from build123d import *

# Parameters (mm, degrees)
F0_W     = 60.3283978999
F0_H     = 56.9055080414
F1_DEPTH = 25.4
F3_DEPTH = 5.08
F5_DEPTH = 25.401


with BuildPart() as f1:
    # F0 (on Top) → F1 (new body)
    with BuildSketch(Plane.XY):
        with Locations((30.1641989499, 28.4527540207)):
            Rectangle(F0_W, F0_H)
    extrude(amount=F1_DEPTH)

    # F2 (on face) → F3 (cut)
    with BuildSketch(Plane.XY.offset(25.4)):
        with BuildLine():
            ThreePointArc((55.1804514534, 39.8446242733), (55.3108318877, 40.8708207203), (55.3543950429, 41.9043488801))
            ThreePointArc((55.3543950429, 41.9043488801), (36.2534657798, 52.11936711), (38.3624892299, 30.5614424362))
            ThreePointArc((38.3624892299, 30.5614424362), (42.0828202021, 43.6972697394), (55.1804514534, 39.8446242733))
        make_face()
        with BuildLine():
            ThreePointArc((55.1804514534, 39.8446242733), (42.0828202021, 43.6972697394), (38.3624892299, 30.5614424362))
            ThreePointArc((38.3624892299, 30.5614424362), (49.0077038635, 31.1517402149), (55.1804514534, 39.8446242733))
        make_face()
        with BuildLine():
            ThreePointArc((55.1804514534, 39.8446242733), (49.0077038635, 31.1517402149), (38.3624892299, 30.5614424362))
            ThreePointArc((38.3624892299, 30.5614424362), (49.1682517649, 25.9984305066), (56.3300997812, 35.287860781))
            ThreePointArc((56.3300997812, 35.287860781), (56.0382540759, 37.6376365577), (55.1804514534, 39.8446242733))
        make_face()
    extrude(amount=-F3_DEPTH, mode=Mode.SUBTRACT)

    # F4 (on face) → F5 (cut, through all)
    with BuildSketch(Plane.XY.offset(25.4)):
        with BuildLine():
            ThreePointArc((37.0080242328, 52.5846074944), (10.3680448546, 12.5437070116), (55.898797074, 28.0328262597))
            ThreePointArc((55.898797074, 28.0328262597), (55.8323251046, 29.8692242337), (55.6332571118, 31.6960104763))
            ThreePointArc((55.6332571118, 31.6960104763), (47.3543007953, 25.7030679225), (38.3624892299, 30.5614424362))
            ThreePointArc((38.3624892299, 30.5614424362), (30.8137212617, 41.1504129454), (37.0080242328, 52.5846074944))
        make_face()
        with BuildLine():
            ThreePointArc((38.3624892299, 30.5614424362), (47.3543007953, 25.7030679225), (55.6332571118, 31.6960104763))
            ThreePointArc((55.6332571118, 31.6960104763), (49.4570170906, 44.9368463083), (37.0080242328, 52.5846074944))
            ThreePointArc((37.0080242328, 52.5846074944), (30.8137212617, 41.1504129454), (38.3624892299, 30.5614424362))
        make_face()
    extrude(amount=-F5_DEPTH, mode=Mode.SUBTRACT)


solid = f1.part
Design review of the part built by this model. Coordinates are the model's own, in mm. Round coordinates to 2 decimals unless told otherwise and drop trailing zeros. Loops run counter-clockwise (first coordinate to the right, second up) from the corner with the lowest first, then second, coordinate; pieces in that order, holes last. Notation, with made-up numbers: M 63,-30 L 102,-30 A9 cw 102,-18 Z; hole C 42.25,67.5 d8. An arc over 180 degrees is marked long. Answer as a JSON object with one key per item and string values.
Item 1: Wall thickness on L1, parallel to X at y = 28, z = 2.75; L2, parallel to Y at x = 31, z = 20.5; L3, parallel to X at y = 30, z = 12.25: over which ranges is each line inside the solid? List them lowest first. Write a range as from..to.
Answer sheet:
{"L1": "x = 0..5.1, 55.9..60.33", "L2": "y = 0..2.64, 53.43..56.91", "L3": "x = 0..5.18, 55.82..60.33"}
Item 2: We need section C-C on x = 17. Give the boundary of the cut face in (y, z).
Answer sheet:
{"outline": "M 0,0 L 6.52,0 L 6.52,25.4 L 0,25.4 Z; M 49.55,0 L 56.91,0 L 56.91,25.4 L 49.55,25.4 Z"}
Item 3: The part is to be moulded in two halves that separate along X. For faces 1 (the flat face through (0, 28, 13)), 2 (the flat face through (30, 54, 25.4)), 3 (the flat face through (49, 47, 20.32)), 4 (the flat face through (60.328, 28, 13)), say which applies: pulls with the +X half, pulls with the -X half, needs draft (parallel to the pull), parting line crosses it, or undercut.
Answer sheet:
{"face 1": "pulls with the -X half", "face 2": "needs draft", "face 3": "undercut", "face 4": "pulls with the +X half"}
Item 4: We need section A-A on z = 13.25. Give the boundary of the cut face in (x, y).
Answer sheet:
{"outline": "M 0,0 L 60.33,0 L 60.33,56.91 L 0,56.91 Z; hole C 30.5,28.03 d50.8"}
Item 5: We need section B-B on y = 48.5. Give the boundary of the cut face in (x, z), and give its area (3 significant figures).
Answer sheet:
{"outline": "M 0,0 L 15.46,0 L 15.46,25.4 L 0,25.4 Z; M 45.54,0 L 60.33,0 L 60.33,25.4 L 53.43,25.4 L 53.43,20.32 L 45.54,20.32 Z", "area": "728 mm^2"}
Item 6: Clearance check with a flat-ended pin moving along its axis: P1, Ø6, axis at x = 48.5, y = 47, coming from the +Z side. State where the tip first meets the part, or that it passes through.
Answer sheet:
{"P1": "stops at z = 20.32"}
Item 7: We need section D-D on y = 23. Give the boundary of the cut face in (x, z), and give its area (3 significant figures).
Answer sheet:
{"outline": "M 0,0 L 5.6,0 L 5.6,25.4 L 0,25.4 Z; M 55.4,0 L 60.33,0 L 60.33,25.4 L 55.4,25.4 Z", "area": "268 mm^2"}
